Can you work these out from the model? Positions are in its coordinate system, mm. Give positions to 0.01 mm unless a question says otherwise; leave off trailing zeros. Loops run counter-clockwise (first coordinate to the right, second up) from the corner with the lowest first, then second, coordinate; pieces in that order, holes last. Notation, with made-up numbers: M 21.25,35 L 50.25,35 A34 ccw 50.25,66 Z; hole C 18.25,43 d5. An arc over 180 degrees is marked long. Answer as a JSON object with one key per item and string values.
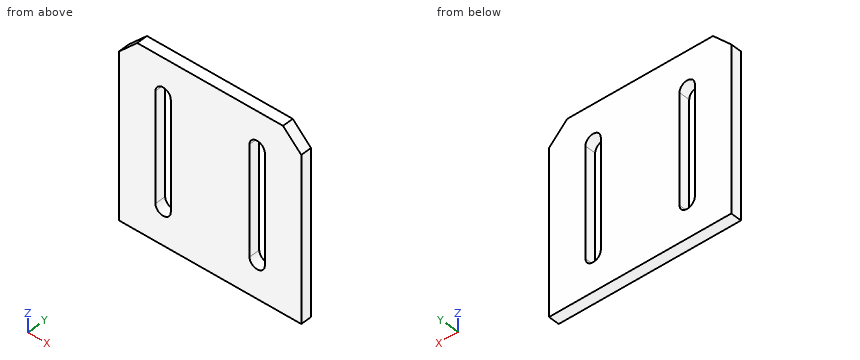
```python
from build123d import *

# Parameters (mm, degrees)
SKETCH1_W           = 50
SKETCH1_H           = 50
BOSS_EXTRUDE1_DEPTH = 3
CHAMFER1_SIZE       = 5
CUT_EXTRUDE1_DEPTH  = 10


with BuildPart() as part:
    # Sketch1 → Boss-Extrude1 (new body)
    with BuildSketch(Plane(origin=(0, 0, 0), x_dir=(1, 0, 0), z_dir=(0, 1, 0))):
        Rectangle(SKETCH1_W, SKETCH1_H)
    extrude(amount=BOSS_EXTRUDE1_DEPTH)

    # Chamfer1
    chamfer1_edges = [part.edges().sort_by_distance(p)[0] for p in [
        (25, 1.5, 25),
        (-25, 1.5, 25),
    ]]
    chamfer(chamfer1_edges, length=CHAMFER1_SIZE)

    # Sketch2 → Cut-Extrude1 (cut)
    with BuildSketch(Plane(origin=(0, 3, 0), x_dir=(1, 0, 0), z_dir=(0, 1, 0))):
        with BuildLine():
            Line((-10.8, -15), (-10.8, 15))
            ThreePointArc((-10.8, 15), (-12.9, 12.9), (-15, 15))
            Line((-15, 15), (-15, -15))
            ThreePointArc((-15, -15), (-12.9, -12.9), (-10.8, -15))
        make_face()
        with BuildLine():
            ThreePointArc((-15, 15), (-12.9, 12.9), (-10.8, 15))
            Line((-10.8, 15), (-15, 15))
        make_face()
        with BuildLine():
            Line((-15, 15), (-10.8, 15))
            ThreePointArc((-10.8, 15), (-12.9, 17.1), (-15, 15))
        make_face()
        with BuildLine():
            ThreePointArc((-15, -15), (-12.9, -17.1), (-10.8, -15))
            Line((-10.8, -15), (-15, -15))
        make_face()
        with BuildLine():
            Line((-15, -15), (-10.8, -15))
            ThreePointArc((-10.8, -15), (-12.9, -12.9), (-15, -15))
        make_face()
        with BuildLine():
            ThreePointArc((15, -15), (12.9, -12.9), (10.8, -15))
            Line((10.8, -15), (15, -15))
        make_face()
        with BuildLine():
            Line((15, -15), (10.8, -15))
            ThreePointArc((10.8, -15), (12.9, -17.1), (15, -15))
        make_face()
        with BuildLine():
            ThreePointArc((15, 15), (12.9, 12.9), (10.8, 15))
            Line((10.8, 15), (10.8, -15))
            ThreePointArc((10.8, -15), (12.9, -12.9), (15, -15))
            Line((15, -15), (15, 15))
        make_face()
        with BuildLine():
            ThreePointArc((15, 15), (12.9, 17.1), (10.8, 15))
            Line((10.8, 15), (15, 15))
        make_face()
        with BuildLine():
            Line((15, 15), (10.8, 15))
            ThreePointArc((10.8, 15), (12.9, 12.9), (15, 15))
        make_face()
    extrude(amount=-CUT_EXTRUDE1_DEPTH, mode=Mode.SUBTRACT)


solid = part.part
```
1) Please list where these lines run through material, in increasing order: line 1 along X through (y, z) = (2, -14); line 2 along Z through (x, y) = (-13, 0.75); line 3 along Z through (x, y) = (12, 1.25). Write a range as from..to.
Answer list:
{"line 1": "-25..-15, -10.8..10.8, 15..25", "line 2": "-25..-17.1, 17.1..25", "line 3": "-25..-16.9, 16.9..25"}
2) Suppose I cut it at C-C, the plane z = -8. Write out the boundary of the cut face in (x, y), and give its area (3 significant figures).
Answer list:
{"outline": "M -25,0 L -15,0 L -15,3 L -25,3 Z; M -10.8,0 L 10.8,0 L 10.8,3 L -10.8,3 Z; M 15,0 L 25,0 L 25,3 L 15,3 Z", "area": "125 mm^2"}
3) Suppose I cut it at B-B, the plane x = 12.9. Write out the boundary of the cut face in (y, z).
Answer list:
{"outline": "M 0,-25 L 3,-25 L 3,-17.1 L 0,-17.1 Z; M 0,17.1 L 3,17.1 L 3,25 L 0,25 Z"}
4) Suppose I cut it at A-A, the plane y = 1.3. Write out the boundary of the cut face in (x, z).
Answer list:
{"outline": "M -25,-25 L 25,-25 L 25,20 L 20,25 L -20,25 L -25,20 Z; hole M -15,-15 A2.1 ccw -10.8,-15 L -10.8,15 A2.1 ccw -15,15 Z; hole M 10.8,-15 A2.1 ccw 15,-15 L 15,15 A2.1 ccw 10.8,15 Z"}
